```python
from build123d import *

# Parameters (mm, degrees)
SKETCH1_W           = 60
SKETCH1_H           = 20
BOSS_EXTRUDE1_DEPTH = 10
CUT_EXTRUDE1_DEPTH  = 7.5
SKETCH5_R           = 2.75
CUT_EXTRUDE3_DEPTH  = 37.827299657
LPATTERN1_COUNT     = 2
LPATTERN1_PITCH     = 17
SKETCH3_R           = 7.5
BOSS_EXTRUDE2_DEPTH = 20
SKETCH4_R           = 3
CUT_EXTRUDE2_DEPTH  = 41.078048855
FILLET1_R           = 10


with BuildPart() as part:
    # Sketch1 → Boss-Extrude1 (new body)
    with BuildSketch(Plane.XY):
        with Locations((0, -10)):
            Rectangle(SKETCH1_W, SKETCH1_H)
    extrude(amount=BOSS_EXTRUDE1_DEPTH)

    # Sketch2 → Cut-Extrude1 (cut)
    with BuildSketch(Plane.XY.offset(10)):
        Polygon((-23.25, -14.907477288), (-19, -12.453738644), (-19, -7.546261356), (-23.25, -5.092522712), (-27.5, -7.546261356), (-27.5, -12.453738644), align=None)
    cut_extrude1 = extrude(amount=-CUT_EXTRUDE1_DEPTH, mode=Mode.SUBTRACT)

    # Sketch5 → Cut-Extrude3 (cut, through all)
    with BuildSketch(Plane.XY.offset(2.5)):
        with Locations((-23.25, -10)):
            Circle(SKETCH5_R)
    cut_extrude3 = extrude(amount=-CUT_EXTRUDE3_DEPTH, mode=Mode.SUBTRACT)

    # LPattern1: Cut-Extrude1, Cut-Extrude3 ×2
    with Locations(*[(i * LPATTERN1_PITCH, 0, 0) for i in range(1, LPATTERN1_COUNT)]):
        add(cut_extrude1, mode=Mode.SUBTRACT)
        add(cut_extrude3, mode=Mode.SUBTRACT)

    # Sketch3 → Boss-Extrude2 (add, through all)
    with BuildSketch(Plane(origin=(0, 0, 0), x_dir=(1, 0, 0), z_dir=(0, 1, 0))):
        with Locations((22.5, -10)):
            Circle(SKETCH3_R)
    extrude(amount=-BOSS_EXTRUDE2_DEPTH)

    # Sketch4 → Cut-Extrude2 (cut, through all)
    with BuildSketch(Plane(origin=(0, 0, 0), x_dir=(1, 0, 0), z_dir=(0, 1, 0))):
        with Locations(Location((22.5, -10, 0), (0, 0, 180))):
            Circle(SKETCH4_R)
    extrude(amount=-CUT_EXTRUDE2_DEPTH, mode=Mode.SUBTRACT)

    # Fillet1
    fillet1_edges = [part.edges().sort_by_distance(p)[0] for p in [
        (15, -10, 10),
    ]]
    fillet(fillet1_edges, radius=FILLET1_R)


solid = part.part
```
Work out the finished part from the listing and answer in its coordinate system (mm). A direction names the side the tool comes from. Round coordinates to 2 decimals unless told otherwise and drop trailing zeros. Loops run counter-clockwise (first coordinate to the right, second up) from the corner with the lowest first, then second, coordinate; pieces in that order, holes last. Notation, with made-up numbers: M -2.75,-35.75 L 9.25,-35.75 A28 cw 9.25,-11.75 Z; hole C 60,69.25 d3. An arc over 180 degrees is marked long. One line per question, with ' | ' between items.
Q1. Consider line 1 along Z through (x, y) = (22.5, -15); line 2 along X through (y, z) = (-6.25, 9.75); line 3 along Y through (x, z) = (-23.25, 0.65). Determine where each line is inside the solid, lowest interval first. Write a range as from..to.
Conclusion:
line 1: z = 0..7, 13..17.5 | line 2: x = -30..-25.25, -21.25..-8.25, -4.25..19.51, 25.49..30 | line 3: y = -20..-12.75, -7.25..0
Q2. Find section A-A, the plane y = -10. Give the vertices of the cut face in (x, z).
Conclusion:
outline: M -30,0 L -26,0 L -26,2.5 L -27.5,2.5 L -27.5,10 L -30,10 Z; M -20.5,0 L -9,0 L -9,2.5 L -10.5,2.5 L -10.5,10 L -19,10 L -19,2.5 L -20.5,2.5 Z; M -3.5,0 L 30,0 L 30,10 A7.5 ccw 16.35,14.29 A10 cw 8.14,10 L -2,10 L -2,2.5 L -3.5,2.5 Z; hole C 22.5,10 d6
Q3. Find section D-D, the plane y = -1.75. Give the vertices of the cut face in (x, z).
Conclusion:
outline: M -30,0 L 30,0 L 30,10 A7.5 ccw 16.35,14.29 A10 cw 8.14,10 L -30,10 Z; hole C 22.5,10 d6
Q4. The mould has two halves that part along X. Classify faces 1 (the cylindrical face through (12.83, -9.86, 11.17)), 2 (the flat face through (-4.095, -6.337, 6.302)), 3 (the flat face through (6, 0, 7)): +X half, -X half, draft (parallel to the pull), parting line (faces both ways), or undercut.
Conclusion:
face 1: -X half | face 2: undercut | face 3: draft
Q5. Find section B-B, the plane x = 22.5. Give the vertices of the cut face in (y, z).
Conclusion:
outline: M -20,0 L 0,0 L 0,7 L -20,7 Z; M -20,13 L 0,13 L 0,17.5 L -20,17.5 Z
Q6. Each of these flat-tipped pins is pushed along its axis until it touches: pin 1 Ø9.5 at (x, y) = (-24.5, -9) entering from +Z; pin 2 Ø8 at (x, y) = (-12.5, -8) entering from -Z; pin 3 Ø3.5 at (x, y) = (-23.25, -10) entering from -Z. Where does it stop, or does it pass through?
Conclusion:
pin 1: stops at z = 10 | pin 2: stops at z = 0 | pin 3: passes through
Q7. A tool of negligible diameter and unlimited length cuts with its end or side. For faces 4 (the flat face through (30, -10, 5)), 5 (the flat face through (-4.155, -13.698, 6.302)), 6 (the flat face through (-11, -10, 10)), from which of +Z, -Z, +X, -X, +Y, -Y can it reach the whole face along a straight path? Write none if from no direction.
Conclusion:
face 4: +Z, -Z, +X, +Y, -Y | face 5: +Z | face 6: +Z, -X, +Y, -Y
Q8. Find section C-C, the plane z = 10.75. Give the vertices of the cut face in (x, y).
Conclusion:
outline: M 11.94,-20 L 19.6,-20 L 19.6,0 L 11.94,0 Z; M 25.4,-20 L 29.96,-20 L 29.96,0 L 25.4,0 Z
